Build history of the part. All positions in model axes, mm. A direction names the side the tool comes from. Round coordinates to 2 decimals unless told otherwise and drop trailing zeros. Loops run counter-clockwise (first coordinate to the right, second up) from the corner with the lowest first, then second, coordinate; pieces in that order, holes last.
from build123d import *

# Parameters (mm, degrees)
SKETCH1_W           = 25
SKETCH1_H           = 25
SKETCH1_W_2         = 23
SKETCH1_H_2         = 23
BOSS_EXTRUDE1_DEPTH = 250
SKETCH3_R           = 2
CUT_EXTRUDE1_DEPTH  = 25
SKETCH4_R           = 2
CUT_EXTRUDE2_DEPTH  = 25
SKETCH5_R           = 2
CUT_EXTRUDE3_DEPTH  = 25


with BuildPart() as part:
    # Sketch1 → Boss-Extrude1 (new body)
    with BuildSketch(Plane(origin=(0, 0, 0), x_dir=(1, 0, 0), z_dir=(0, 1, 0))):
        Rectangle(SKETCH1_W, SKETCH1_H)
        Rectangle(SKETCH1_W_2, SKETCH1_H_2, mode=Mode.SUBTRACT)
    extrude(amount=BOSS_EXTRUDE1_DEPTH)

    # Sketch3 → Cut-Extrude1 (cut)
    with BuildSketch(Plane(origin=(12.5, 0, 0), x_dir=(0, 0, -1), z_dir=(1, 0, 0))):
        with Locations((7.5, 245)):
            Circle(SKETCH3_R)
        with Locations((7.5, 235)):
            Circle(SKETCH3_R)
        with Locations((-7.5, 245)):
            Circle(SKETCH3_R)
        with Locations((-7.5, 235)):
            Circle(SKETCH3_R)
        with Locations((7.5, 225)):
            Circle(SKETCH3_R)
        with Locations((-7.5, 225)):
            Circle(SKETCH3_R)
    extrude(amount=-CUT_EXTRUDE1_DEPTH, mode=Mode.SUBTRACT)

    # Sketch4 → Cut-Extrude2 (cut)
    with BuildSketch(Plane.XY.offset(12.5)):
        with Locations((5.5, 218)):
            Circle(SKETCH4_R)
        with Locations((5.5, 207)):
            Circle(SKETCH4_R)
    cut_extrude2 = extrude(amount=-CUT_EXTRUDE2_DEPTH, mode=Mode.SUBTRACT)

    # Sketch5 → Cut-Extrude3 (cut)
    with BuildSketch(Plane.XY.offset(12.5)):
        with Locations((0, 12.5)):
            Circle(SKETCH5_R)
    extrude(amount=-CUT_EXTRUDE3_DEPTH, mode=Mode.SUBTRACT)

    # Mirror1: Cut-Extrude2 across plane
    add(cut_extrude2.mirror(Plane(origin=(0, 0, 0), x_dir=(0, 0, 1), z_dir=(1, 0, 0))), mode=Mode.SUBTRACT)


solid = part.part
(1) Pull direction Y, two halves, no side cores. Call faces 1 (the face through (0, 123, -11.5)), 2 (the face through (-1, 0, 12)), 3 (the face through (12.007, 233.226, -8.423)): +Y half, -Y half, draft (parallel to the pull), parting line (faces both ways), or undercut.
Responses:
face 1: draft
face 2: -Y half
face 3: undercut
(2) Which spindle directions (+Z, -Z, +X, -X, +Y, -Y) get a long thin tool onto all of the face, cutting with end or side? Do faces 4 (the face through (0, 123, 11.5)), 5 (the face through (12.007, 243.226, -8.423)). Say none if no direction does.
Responses:
face 4: +Y, -Y
face 5: +X, -X
(3) Probe line 1 (Z direction, x = 12.1, y = 245); line 2 (Y direction, x = 5.5, z = -11.95); line 3 (Y direction, x = -11.65, z = 7.5). List the from-to ranges inside material, lowest first.
Responses:
line 1: z = -12.5 to -9.5, -5.5 to 5.5, 9.5 to 12.5
line 2: y = 0 to 205, 209 to 216, 220 to 250
line 3: y = 0 to 223, 227 to 233, 237 to 243, 247 to 250
(4) Slice it at B-B on y = 107. List the corners of the cut face in (x, z), plus the area to 3 significant figures.
Responses:
outline: (-12.5, -12.5) - (12.5, -12.5) - (12.5, 12.5) - (-12.5, 12.5) - close; hole (-11.5, -11.5) - (11.5, -11.5) - (11.5, 11.5) - (-11.5, 11.5) - close
area: 96.0 mm2
(5) Slice it at A-A on z = 3. List the corners of the cut face in (x, y).
Responses:
outline: (-12.5, 0) - (-11.5, 0) - (-11.5, 250) - (-12.5, 250) - close; (11.5, 0) - (12.5, 0) - (12.5, 250) - (11.5, 250) - close
